CAD build for the part. Positions are in the model's coordinates, mm. A direction names the side the tool comes from. Give positions to 0.01 mm unless a question says otherwise; leave off trailing zeros. Write each loop counter-clockwise with the first axis right and the second up, starting at its lowest first coordinate (ties: lowest second). Pieces come first, ordered by that corner, then holes. Notation, with made-up numbers: (-8, -33.75) -> (11, -33.75) arc R26 cw to (11, -14.75) -> close; hole circle Ø2 at (-39.75, -3). An arc over 180 degrees is marked (long way). Answer as a JSON object with one key per item and string values.
```python
from build123d import *

# Parameters (mm, degrees)
SKETCH_1_W          = 52
SKETCH_1_H          = 70
EXTRUDE_1_DEPTH     = 12
SKETCH_2_R          = 3
CUT_EXTRUDE_1_DEPTH = 10
CUT_EXTRUDE_START   = -10
SKETCH_3_R          = 3
CUT_EXTRUDE_2_DEPTH = 10
SKETCH_4_R          = 3
CUT_EXTRUDE_3_DEPTH = 12


with BuildPart() as part:
    # 草图1 → 凸台-拉伸1 (new body)
    with BuildSketch(Plane.XY):
        Rectangle(SKETCH_1_W, SKETCH_1_H)
    extrude(amount=EXTRUDE_1_DEPTH)

    # 草图2 → 切除-拉伸1 (cut)
    with BuildSketch(Plane.ZY.offset(26)):
        with Locations((6, 27)):
            Circle(SKETCH_2_R)
        with Locations((6, 9)):
            Circle(SKETCH_2_R)
        with Locations((6, -9)):
            Circle(SKETCH_2_R)
        with Locations((6, -27)):
            Circle(SKETCH_2_R)
    extrude(amount=-CUT_EXTRUDE_1_DEPTH, mode=Mode.SUBTRACT)

    # 草图3 → 切除-拉伸2 (cut)
    with BuildSketch(Plane(origin=(26, 0, 0), x_dir=(0, 0, -1), z_dir=(1, 0, 0)).offset(CUT_EXTRUDE_START)):
        with Locations(Location((-6, 27, 0), (0, 0, 180))):
            Circle(SKETCH_3_R)
        with Locations(Location((-6, 9, 0), (0, 0, 180))):
            Circle(SKETCH_3_R)
        with Locations(Location((-6, -9, 0), (0, 0, 180))):
            Circle(SKETCH_3_R)
        with Locations(Location((-6, -27, 0), (0, 0, 180))):
            Circle(SKETCH_3_R)
    extrude(amount=CUT_EXTRUDE_2_DEPTH, mode=Mode.SUBTRACT)

    # 草图4 → 切除-拉伸3 (cut)
    with BuildSketch(Plane.XY.offset(12)):
        with Locations((16, 0)):
            Circle(SKETCH_4_R)
        with Locations((11.313708499, -11.313708499)):
            Circle(SKETCH_4_R)
        with Locations((0, -16)):
            Circle(SKETCH_4_R)
        with Locations((-11.313708499, -11.313708499)):
            Circle(SKETCH_4_R)
        with Locations((-16, 0)):
            Circle(SKETCH_4_R)
        with Locations((-11.313708499, 11.313708499)):
            Circle(SKETCH_4_R)
        with Locations((0, 16)):
            Circle(SKETCH_4_R)
        with Locations((11.313708499, 11.313708499)):
            Circle(SKETCH_4_R)
    extrude(amount=-CUT_EXTRUDE_3_DEPTH, mode=Mode.SUBTRACT)


solid = part.part
```
1) Mould opens along Z. For faces 4 (the cylindrical face through (-14.31, -11.18, 6.08)), 5 (the cylindrical face through (20.93, -25.85, 8.77)), 6 (the flat face through (0, 0, 12)), 7 (the flat face through (-16, -27, 6)) say: released by +Z, released by -Z, zero draft, split by the parting line, or undercut.
Model answer:
{"face 4": "zero draft", "face 5": "undercut", "face 6": "released by +Z", "face 7": "undercut"}
2) Slice it at A-A (x = 0). List the corners of the cut face in (y, z).
Model answer:
{"outline": "(-35, 0) -> (-19, 0) -> (-19, 12) -> (-35, 12) -> close; (-13, 0) -> (13, 0) -> (13, 12) -> (-13, 12) -> close; (19, 0) -> (35, 0) -> (35, 12) -> (19, 12) -> close"}
3) Slice it at C-C (y = 16). List the corners of the cut face in (x, z).
Model answer:
{"outline": "(-26, 0) -> (-3, 0) -> (-3, 12) -> (-26, 12) -> close; (3, 0) -> (26, 0) -> (26, 12) -> (3, 12) -> close"}
4) Slice it at B-B (y = 0). List the corners of the cut face in (x, z).
Model answer:
{"outline": "(-26, 0) -> (-19, 0) -> (-19, 12) -> (-26, 12) -> close; (-13, 0) -> (13, 0) -> (13, 12) -> (-13, 12) -> close; (19, 0) -> (26, 0) -> (26, 12) -> (19, 12) -> close"}
5) Pin check, flat tips, straight feed: pin 1 (3.5 mm diameter, centred on y = -9, z = 6, fed in from -X); pin 2 (3.5 mm diameter, centred on y = 27, z = 6, fed in from +X). Stop position of each tip, or through.
Model answer:
{"pin 1": "stops at x = -16", "pin 2": "stops at x = 16"}
6) 3-axis set-ups, long thin cutter, end or side, ignore diameter. For faces 1 (the cylindrical face through (20.93, 6.47, 7.61)), 2 (the flat face through (-16, 27, 6)), 3 (the cylindrical face through (12.698, 8.652, 6.084)): which of +Z, -Z, +X, -X, +Y, -Y reach the whole face in a straight line?
Model answer:
{"face 1": "+X", "face 2": "-X", "face 3": "+Z, -Z"}
7) Wall check: probe 1 along Y at (x, z) = (20.5, 6); probe 2 along Z at (x, y) = (18, -9); probe 3 along X at (y, z) = (-10, 10.25). Give the ranges that are in metal, low to high.
Model answer:
{"probe 1": "y = -35 to -30, -24 to -12, -6 to 6, 12 to 24, 30 to 35", "probe 2": "z = 0 to 3, 9 to 12", "probe 3": "x = -26 to -14.01, -8.62 to 8.62, 14.01 to 26"}
8) Slice it at D-D (z = 1.25). State how many separate pieces and enclosed holes the cut face has, then the cut area to 3 significant figures.
Model answer:
{"separate pieces": "1", "enclosed holes": "8", "area": "3,410 mm2"}
